Autodesk Inventor part; units mm, degrees
ref_plane "YZ Plane" through (0, 0, 0) normal (1, 0, 0) x (0, 1, 0)
ref_plane "XZ Plane" through (0, 0, 0) normal (0, 1, 0) x (-1, 0, 0)
ref_plane "XY Plane" through (0, 0, 0) normal (0, 0, 1) x (1, 0, 0)
sketch "Sketch1" plane through (0, 0, 0) normal (0, 0, 1) x (1, 0, 0)
  line L0 (0, 0) -> (50.8, 0)
  line L1 (50.8, 0) -> (50.8, 139.7)
  line L2 (50.8, 139.7) -> (0, 139.7)
  line L3 (0, 139.7) -> (0, 0)
  dimension "d0" = 50.8
  dimension "d1" = 139.7
extrude "Plate1" add sketch "Sketch1" along normal blind 3.048
fillet "Corner Round1" radius 25.4 1 edges at (50.8, 139.7, 1.524)
fillet "Corner Round1" radius 25.4 1 edges at (0, 139.7, 1.524)
fillet "Corner Round2" radius 12.7 2 edges at (50.8, 0, 1.524) (0, 0, 1.524)
sketch "Sketch2" plane through (0, 0, 0) normal (0, 0, -1) x (-1, 0, 0)
  arc A0 (-20.4, 99.125) -> (-20.4, 123.125) centre (-25.4, 111.125) ccw
  line L0 (-20.4, 123.125) -> (-30.4, 123.125)
  line L1 (-30.4, 99.125) -> (-20.4, 99.125)
  arc A1 (-30.4, 123.125) -> (-30.4, 99.125) centre (-25.4, 111.125) ccw
  circle A2 centre (-13.0256, 98.7506) radius 1.65
  circle A3 centre (-37.7744, 123.4994) radius 1.65
  circle A4 centre (-13.0256, 123.4994) radius 1.65
  circle A5 centre (-37.7744, 98.7506) radius 1.65
  point P0 (0, 0)
extrude "Extrusion1" cut sketch "Sketch2" against normal up to surface (3.048 mm away)
sketch "Sketch3" plane through (0, 0, 3.048) normal (0, 0, 1) x (1, 0, 0)
  circle A0 centre (12.7, 76.2) radius 2.9337
  circle A1 centre (38.1, 76.2) radius 2.9337
  circle A2 centre (38.1, 44.45) radius 2.9337
  circle A3 centre (12.7, 44.45) radius 2.9337
  circle A4 centre (12.7, 12.7) radius 2.9337
  circle A5 centre (38.1, 12.7) radius 2.9337
  circle A6 centre (12.7, 12.7) radius 2.9337
  point P0 (0, 0)
extrude "Extrusion2" cut sketch "Sketch3" against normal up to surface (3.048 mm away)
equation "\"d10\" = Thickness"
equation "\"BendRadius\" = Thickness"
equation "\"BendReliefWidth\" = Thickness"
equation "\"BendReliefDepth\" = 0.5 * Thickness"
equation "\"CornerReliefSize\" = 4 * Thickness"
equation "\"MinimumRemnant\" = 2 * Thickness"
equation "\"TransitionRadius\" = BendRadius"
equation "\"JacobiRadiusSize\" = Thickness"
equation "\"GapSize\" = Thickness"
equation "\"d2\" = BendRadius"
properties part number "pG188Mount"
Can you work these out from the model? Positions are in its coordinate system, mm. A direction names the side the tool comes from. Coordinates: 2 decimals unless noted, no trailing zeros. Loops run counter-clockwise (first coordinate to the right, second up) from the corner with the lowest first, then second, coordinate; pieces in that order, holes last. Notation, with made-up numbers: (-31.75, 79.25) -> (14.25, 79.25) arc R33 cw to (14.25, 110.25) -> close; hole circle Ø6 at (77.25, -1.75). An arc over 180 degrees is marked (long way). Answer as a JSON object with one key per item and string values.
1) Imagine slicing it at C-C (x = 6). Please give me the cut outline in (y, z).
Results:
{"outline": "(1.91, 0) -> (130.7, 0) -> (130.7, 3.05) -> (1.91, 3.05) -> close"}
2) For faces 1 (the face through (25, 99.125, 2)), 2 (the face through (7.64, 132.46, 1.55)), which set-ups out of +Z, -Z, +X, -X, +Y, -Y let a thin tool reach every point of the face, with its end or its side?
Results:
{"face 1": "+Z, -Z", "face 2": "+Z, -Z, -X, +Y"}
3) Thinking about a two-plate mould opening in X: for faces 3 (the face through (38.4, 111.3, 1.5)), 4 (the face through (25, 71, 3.048)), 5 (the face through (36.25, 98.12, 1.5)), 6 (the face through (46.98, 3.62, 1.55)), which applies, pulls with the +X half, pulls with the -X half, needs draft (parallel to the pull), parting line crosses it, or undercut?
Results:
{"face 3": "undercut", "face 4": "needs draft", "face 5": "undercut", "face 6": "pulls with the +X half"}
4) Imagine slicing it at B-B (x = 18.5). Please give me the cut outline in (y, z), then the cut area to 3 significant figures.
Results:
{"outline": "(0, 0) -> (100.11, 0) -> (100.11, 3.05) -> (0, 3.05) -> close; (122.14, 0) -> (138.74, 0) -> (138.74, 3.05) -> (122.14, 3.05) -> close", "area": "356 mm^2"}
5) Imagine slicing it at D-D (x = 47). Please give me the cut outline in (y, z).
Results:
{"outline": "(3.64, 0) -> (127.66, 0) -> (127.66, 3.05) -> (3.64, 3.05) -> close"}
6) For P1, Ø4.5, axis at x = 37.77, y = 123.5, coming from the -Z side, with a flat end and sliding along its axis, tell me the tip position at first contact or that it passes through.
Results:
{"P1": "stops at z = 0"}
7) Imagine slicing it at A-A (y = 44.45). Please give me the cut outline in (x, z).
Results:
{"outline": "(0, 0) -> (9.77, 0) -> (9.77, 3.05) -> (0, 3.05) -> close; (15.63, 0) -> (35.17, 0) -> (35.17, 3.05) -> (15.63, 3.05) -> close; (41.03, 0) -> (50.8, 0) -> (50.8, 3.05) -> (41.03, 3.05) -> close"}
8) If I drill on line 1 (X direction, y = 76, z = 1.6); line 2 (Y direction, x = 10, z = 1.1); line 3 (Y direction, x = 40, z = 1.45), over which ranges is the centre line in solid material (lowest first)?
Results:
{"line 1": "x = 0 to 9.77, 15.63 to 35.17, 41.03 to 50.8", "line 2": "y = 0.29 to 11.55, 13.85 to 43.3, 45.6 to 75.05, 77.35 to 134.5", "line 3": "y = 0.14 to 10.46, 14.94 to 42.21, 46.69 to 73.96, 78.44 to 135.08"}
